Check sheet for the modelled part. Datum: model origin and axes. Units: mm. Coordinates: 2 decimals unless noted, no trailing zeros. Order: outer loops, then holes, each group sorted by start corner. A loop starts at its lowest first (then second) coordinate and runs counter-clockwise, first axis right, second up.
from build123d import *

# Parameters (mm, degrees)
SKETCH_1_R      = 13.5
SKETCH_1_R_2    = 1.55
EXTRUDE_1_DEPTH = 5


with BuildPart() as part:
    # 草图1 → 凸台-拉伸1 (new body)
    with BuildSketch(Plane(origin=(0, 0, 0), x_dir=(1, 0, 0), z_dir=(0, 1, 0))):
        with BuildLine():
            Line((-49, 21), (49, 21))
            ThreePointArc((49, 21), (70, 0), (49, -21))
            Line((49, -21), (-49, -21))
            ThreePointArc((-49, -21), (-70, 0), (-49, 21))
        make_face()
        with Locations(Location((-49, 0, 0), (0, 0, 270))):
            Circle(SKETCH_1_R, mode=Mode.SUBTRACT)
        with Locations(Location((-49, 17.5, 0), (0, 0, 270))):
            Circle(SKETCH_1_R_2, mode=Mode.SUBTRACT)
        with Locations(Location((-20, 13, 0), (0, 0, 270))):
            Circle(SKETCH_1_R_2, mode=Mode.SUBTRACT)
        with Locations(Location((-20, -13, 0), (0, 0, 270))):
            Circle(SKETCH_1_R_2, mode=Mode.SUBTRACT)
        with Locations(Location((-40.25, 15.155444566, 0), (0, 0, 270))):
            Circle(SKETCH_1_R_2, mode=Mode.SUBTRACT)
        with Locations(Location((-33.844555434, 8.75, 0), (0, 0, 270))):
            Circle(SKETCH_1_R_2, mode=Mode.SUBTRACT)
        with Locations(Location((-31.5, 0, 0), (0, 0, 270))):
            Circle(SKETCH_1_R_2, mode=Mode.SUBTRACT)
        with Locations(Location((-33.844555434, -8.75, 0), (0, 0, 270))):
            Circle(SKETCH_1_R_2, mode=Mode.SUBTRACT)
        with Locations(Location((-40.25, -15.155444566, 0), (0, 0, 270))):
            Circle(SKETCH_1_R_2, mode=Mode.SUBTRACT)
        with Locations(Location((-49, -17.5, 0), (0, 0, 270))):
            Circle(SKETCH_1_R_2, mode=Mode.SUBTRACT)
        with Locations(Location((-57.75, -15.155444566, 0), (0, 0, 270))):
            Circle(SKETCH_1_R_2, mode=Mode.SUBTRACT)
        with Locations(Location((-64.155444566, -8.75, 0), (0, 0, 270))):
            Circle(SKETCH_1_R_2, mode=Mode.SUBTRACT)
        with Locations(Location((-66.5, 0, 0), (0, 0, 270))):
            Circle(SKETCH_1_R_2, mode=Mode.SUBTRACT)
        with Locations(Location((-64.155444566, 8.75, 0), (0, 0, 270))):
            Circle(SKETCH_1_R_2, mode=Mode.SUBTRACT)
        with Locations(Location((-57.75, 15.155444566, 0), (0, 0, 270))):
            Circle(SKETCH_1_R_2, mode=Mode.SUBTRACT)
        with Locations(Location((57.75, 15.155444566, 0), (0, 0, 90))):
            Circle(SKETCH_1_R_2, mode=Mode.SUBTRACT)
        with Locations(Location((64.155444566, 8.75, 0), (0, 0, 90))):
            Circle(SKETCH_1_R_2, mode=Mode.SUBTRACT)
        with Locations(Location((66.5, 0, 0), (0, 0, 90))):
            Circle(SKETCH_1_R_2, mode=Mode.SUBTRACT)
        with Locations(Location((64.155444566, -8.75, 0), (0, 0, 90))):
            Circle(SKETCH_1_R_2, mode=Mode.SUBTRACT)
        with Locations(Location((57.75, -15.155444566, 0), (0, 0, 90))):
            Circle(SKETCH_1_R_2, mode=Mode.SUBTRACT)
        with Locations(Location((49, -17.5, 0), (0, 0, 90))):
            Circle(SKETCH_1_R_2, mode=Mode.SUBTRACT)
        with Locations(Location((40.25, -15.155444566, 0), (0, 0, 90))):
            Circle(SKETCH_1_R_2, mode=Mode.SUBTRACT)
        with Locations(Location((33.844555434, -8.75, 0), (0, 0, 90))):
            Circle(SKETCH_1_R_2, mode=Mode.SUBTRACT)
        with Locations(Location((31.5, 0, 0), (0, 0, 90))):
            Circle(SKETCH_1_R_2, mode=Mode.SUBTRACT)
        with Locations(Location((40.25, 15.155444566, 0), (0, 0, 90))):
            Circle(SKETCH_1_R_2, mode=Mode.SUBTRACT)
        with Locations(Location((20, -13, 0), (0, 0, 90))):
            Circle(SKETCH_1_R_2, mode=Mode.SUBTRACT)
        with Locations(Location((20, 13, 0), (0, 0, 90))):
            Circle(SKETCH_1_R_2, mode=Mode.SUBTRACT)
        with Locations(Location((49, 17.5, 0), (0, 0, 90))):
            Circle(SKETCH_1_R_2, mode=Mode.SUBTRACT)
        with Locations(Location((49, 0, 0), (0, 0, 90))):
            Circle(SKETCH_1_R, mode=Mode.SUBTRACT)
        with Locations(Location((33.844555434, 8.75, 0), (0, 0, 90))):
            Circle(SKETCH_1_R_2, mode=Mode.SUBTRACT)
    extrude(amount=EXTRUDE_1_DEPTH)


solid = part.part
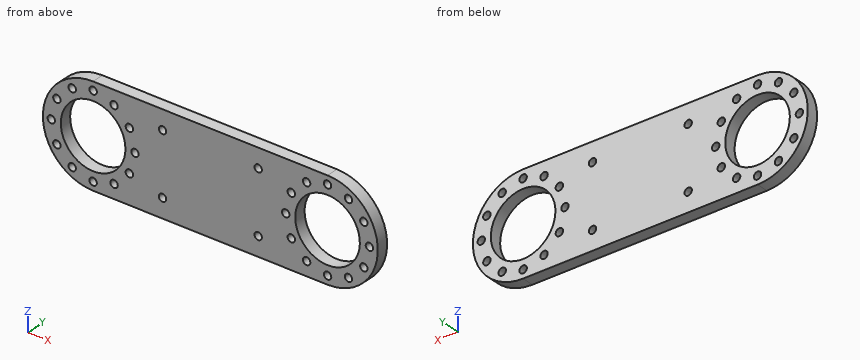
(1) Cross-section at C-C (y = 1.4). Count the separate pieces of the cut face and the enclosed holes in it, and give its area (4 significant figures).
Filled in:
separate pieces: 1
enclosed holes: 30
area: 4,145 mm2
(2) Cross-section at D-D (x = 43). Enter the section's corners in (y, z).
Filled in:
outline: (0, -21) - (5, -21) - (5, -12.09) - (0, -12.09) - close; (0, 12.09) - (5, 12.09) - (5, 21) - (0, 21) - close
(3) Thickness scan on probe 1 along Z at (x, y) = (49, 2.75); probe 2 along X at (y, z) = (2.7, 3.5); probe 3 along Z at (x, y) = (-50, 0.85). Record the ranges inside material, lowest first.
Filled in:
probe 1: z = -21 to -19.05, -15.95 to -13.5, 13.5 to 15.95, 19.05 to 21
probe 2: x = -69.71 to -62.04, -35.96 to 35.96, 62.04 to 69.71
probe 3: z = -20.98 to -18.68, -16.32 to -13.46, 13.46 to 16.32, 18.68 to 20.98
(4) Cross-section at B-B (z = 8.75). Enter the section's corners in (x, y), and give its area (3 significant figures).
Filled in:
outline: (-68.09, 0) - (-65.71, 0) - (-65.71, 5) - (-68.09, 5) - close; (-62.61, 0) - (-59.28, 0) - (-59.28, 5) - (-62.61, 5) - close; (-38.72, 0) - (-35.39, 0) - (-35.39, 5) - (-38.72, 5) - close; (-32.29, 0) - (32.29, 0) - (32.29, 5) - (-32.29, 5) - close; (35.39, 0) - (38.72, 0) - (38.72, 5) - (35.39, 5) - close; (59.28, 0) - (62.61, 0) - (62.61, 5) - (59.28, 5) - close; (65.71, 0) - (68.09, 0) - (68.09, 5) - (65.71, 5) - close
area: 413 mm2
(5) Cross-section at A-A (x = 20). Enter the section's corners in (y, z), and give its area (3 significant figures).
Filled in:
outline: (0, -21) - (5, -21) - (5, -14.55) - (0, -14.55) - close; (0, -11.45) - (5, -11.45) - (5, 11.45) - (0, 11.45) - close; (0, 14.55) - (5, 14.55) - (5, 21) - (0, 21) - close
area: 179 mm2
(6) Go/stop test with flat-tipped pins: P1, Ø4, axis at x = -66.5, z = 0, coming from the -Y side; P2, Ø1.9, axis at x = -20, z = -13, coming from the -Y side; P3, Ø1.5, axis at y = 1.5, z = -4, coming from the -X side. Record where each tip stops, or that it passes through.
Filled in:
P1: stops at y = 0
P2: passes through
P3: stops at x = -69.75
